The model under review builds one solid part; all positions refer to its coordinate system, in mm. Round coordinates to 2 decimals unless told otherwise and drop trailing zeros. Order: outer loops, then holes, each group sorted by start corner. A loop starts at its lowest first (then second) coordinate and runs counter-clockwise, first axis right, second up. Notation, with made-up numbers: M 71,-28 L 118,-28 A27 cw 118,1 Z; hole C 79.5,20 d6. An arc over 180 degrees is marked long. Answer as a JSON object with one key per item and string values. Group by question number.
1. To check wall thickness, follow probe 1 along Y at (x, z) = (-138.5, 4). State the ranges of the line that lie inside material, in increasing order. Write a range as [from, to].
2. Clearance check with a flat-ended pin moving along its axis: P1, Ø10, axis at x = -90, y = 12, coming from the -Z side. State where the tip first meets the part, or that it passes through.
3. Add section B-B on x = 138.5. State the section outline as (y, z) points.
4. Mouldability with a two-part tool opening along Y and no side actions: class faces 1 (the face through (141.502, -46.245, 5.423)), 2 (the face through (-2, 75, 5)), 3 (the face through (-2, -75, 5)) as released by +Y, released by -Y, zero draft, split by the parting line, or undercut.
5. Add section A-A on y = 45. State the section outline as (x, z) points.
```python
from build123d import *

# Parameters (mm, degrees)
SKETCH2_W           = 317
SKETCH2_H           = 150
SKETCH2_R           = 3.25
BOSS_EXTRUDE1_DEPTH = 11


with BuildPart() as part:
    # Sketch2 → Boss-Extrude1 (new body)
    with BuildSketch(Plane.XY):
        Rectangle(SKETCH2_W, SKETCH2_H)
        with Locations((-138.5, 45)):
            Circle(SKETCH2_R, mode=Mode.SUBTRACT)
        with Locations(Location((138.5, 45, 0), (0, 0, 180))):
            Circle(SKETCH2_R, mode=Mode.SUBTRACT)
        with Locations((138.5, -45)):
            Circle(SKETCH2_R, mode=Mode.SUBTRACT)
        with Locations(Location((-138.5, -45, 0), (0, 0, 180))):
            Circle(SKETCH2_R, mode=Mode.SUBTRACT)
    extrude(amount=BOSS_EXTRUDE1_DEPTH)


solid = part.part
```
Recorded:
{
 "1": {"probe 1": "y = [-75, -48.25], [-41.75, 41.75], [48.25, 75]"},
 "2": {"P1": "stops at z = 0"},
 "3": {"outline": "M -75,0 L -48.25,0 L -48.25,11 L -75,11 Z; M -41.75,0 L 41.75,0 L 41.75,11 L -41.75,11 Z; M 48.25,0 L 75,0 L 75,11 L 48.25,11 Z"},
 "4": {"face 1": "undercut", "face 2": "released by +Y", "face 3": "released by -Y"},
 "5": {"outline": "M -158.5,0 L -141.75,0 L -141.75,11 L -158.5,11 Z; M -135.25,0 L 135.25,0 L 135.25,11 L -135.25,11 Z; M 141.75,0 L 158.5,0 L 158.5,11 L 141.75,11 Z"}
}
